```python
from build123d import *

# Parameters (mm, degrees)
ESQUISSE1_R             = 6.5
BOSS_EXTRU_1_DEPTH      = 1
ESQUISSE2_R             = 4.75
BOSS_EXTRU_2_DEPTH      = 6.2
ESQUISSE3_R             = 6.5
BOSS_EXTRU_3_DEPTH      = 1
ESQUISSE4_R             = 1.5
ENL_V_MAT_EXTRU_1_DEPTH = 10


with BuildPart() as part:
    # Esquisse1 → Boss.-Extru.1 (new body)
    with BuildSketch(Plane.XY):
        Circle(ESQUISSE1_R)
    extrude(amount=BOSS_EXTRU_1_DEPTH)

    # Esquisse2 → Boss.-Extru.2 (add)
    with BuildSketch(Plane.XY.offset(1)):
        with Locations(Location((0, 0, 0), (0, 0, 180))):
            Circle(ESQUISSE2_R)
    extrude(amount=BOSS_EXTRU_2_DEPTH)

    # Esquisse3 → Boss.-Extru.3 (add)
    with BuildSketch(Plane.XY.offset(7.2)):
        Circle(ESQUISSE3_R)
    extrude(amount=BOSS_EXTRU_3_DEPTH)

    # Esquisse4 → Enlèv. mat.-Extru.1 (cut)
    with BuildSketch(Plane.XY.offset(8.2)):
        Circle(ESQUISSE4_R)
    extrude(amount=-ENL_V_MAT_EXTRU_1_DEPTH, mode=Mode.SUBTRACT)


solid = part.part
```
Model file for the job. Use its own axes, mm. A direction names the side the tool comes from. Coordinates: 2 decimals unless noted, no trailing zeros. Order: outer loops, then holes, each group sorted by start corner. A loop starts at its lowest first (then second) coordinate and runs counter-clockwise, first axis right, second up. Notation, with made-up numbers: (-34, 55) -> (-20, 55) arc R28 ccw to (-20, 90) -> close; hole circle Ø7 at (5.5, 58). An arc over 180 degrees is marked (long way). Return JSON: item names as keys, results as strings.
Item 1: Wall check: line 1 along Y through (x, z) = (0, 6); line 2 along Z through (x, y) = (-4.25, -4); line 3 along Y through (x, z) = (-0.75, 6.25). Give the ranges that are in metal, low to high. Write a range as from..to.
Model answer:
{"line 1": "y = -4.75..-1.5, 1.5..4.75", "line 2": "z = 0..1, 7.2..8.2", "line 3": "y = -4.69..-1.3, 1.3..4.69"}
Item 2: Pin check, flat tips, straight feed: P1, Ø1.5, axis at y = -4.5, z = 6, coming from the -X side; P2, Ø1.5, axis at x = -2.5, z = 4.5, coming from the -Y side; P3, Ø1.8, axis at x = 0, y = 0, coming from the +Z side. Stop position of each tip, or through.
Model answer:
{"P1": "stops at x = -2.92", "P2": "stops at y = -4.42", "P3": "passes through"}
Item 3: 3-axis set-ups, long thin cutter, end or side, ignore diameter. For faces 4 (the face through (1.03, 4.637, 4.057)), 5 (the face through (0, 2, 8.2)): which of +Z, -Z, +X, -X, +Y, -Y reach the whole face in a straight line?
Model answer:
{"face 4": "none", "face 5": "+Z, +X, -X, +Y, -Y"}
Item 4: Mould opens along X. For faces 1 (the face through (-5.158, -3.955, 7.693)), 2 (the face through (-1.5, 0.07, 4.16)), 3 (the face through (0, -5, 1)) say: pulls with the +X half, pulls with the -X half, needs draft (parallel to the pull), parting line crosses it, or undercut.
Model answer:
{"face 1": "parting line crosses it", "face 2": "undercut", "face 3": "needs draft"}
Item 5: Slice it at B-B (y = -5.25). Write the cut outline in (x, z), then the cut area to 3 significant figures.
Model answer:
{"outline": "(-3.83, 0) -> (3.83, 0) -> (3.83, 1) -> (-3.83, 1) -> close; (-3.83, 7.2) -> (3.83, 7.2) -> (3.83, 8.2) -> (-3.83, 8.2) -> close", "area": "15.3 mm²"}
Item 6: Slice it at A-A (x = 0). Write the cut outline in (y, z), then the cut area to 3 significant figures.
Model answer:
{"outline": "(-6.5, 0) -> (-1.5, 0) -> (-1.5, 8.2) -> (-6.5, 8.2) -> (-6.5, 7.2) -> (-4.75, 7.2) -> (-4.75, 1) -> (-6.5, 1) -> close; (1.5, 0) -> (6.5, 0) -> (6.5, 1) -> (4.75, 1) -> (4.75, 7.2) -> (6.5, 7.2) -> (6.5, 8.2) -> (1.5, 8.2) -> close", "area": "60.3 mm²"}
Item 7: Slice it at D-D (x = 1.75). Write the cut outline in (y, z), then the cut area to 3 significant figures.
Model answer:
{"outline": "(-6.26, 0) -> (6.26, 0) -> (6.26, 1) -> (4.42, 1) -> (4.42, 7.2) -> (6.26, 7.2) -> (6.26, 8.2) -> (-6.26, 8.2) -> (-6.26, 7.2) -> (-4.42, 7.2) -> (-4.42, 1) -> (-6.26, 1) -> close", "area": "79.8 mm²"}
Item 8: Slice it at C-C (z = 2.5). Write the cut outline in (x, y), then the cut area to 3 significant figures.
Model answer:
{"outline": "circle Ø9.5 at (0, 0); hole circle Ø3 at (0, 0)", "area": "63.8 mm²"}
